For this review, use the dimensioned drawing (mm, ordinates from the lowest corner) and the shaded views. A direction names the side the tool comes from. Round coordinates to 2 decimals unless told otherwise and drop trailing zeros. Order: outer loops, then holes, each group sorted by start corner. A loop starts at its lowest first (then second) coordinate and runs counter-clockwise, first axis right, second up. Notation, with made-up numbers: M 63,26 L 105,26 A27 ccw 105,42 Z; hole C 63,-15 d2. An arc over 180 degrees is marked long. One line per item, written item: value. Start each with the question number.
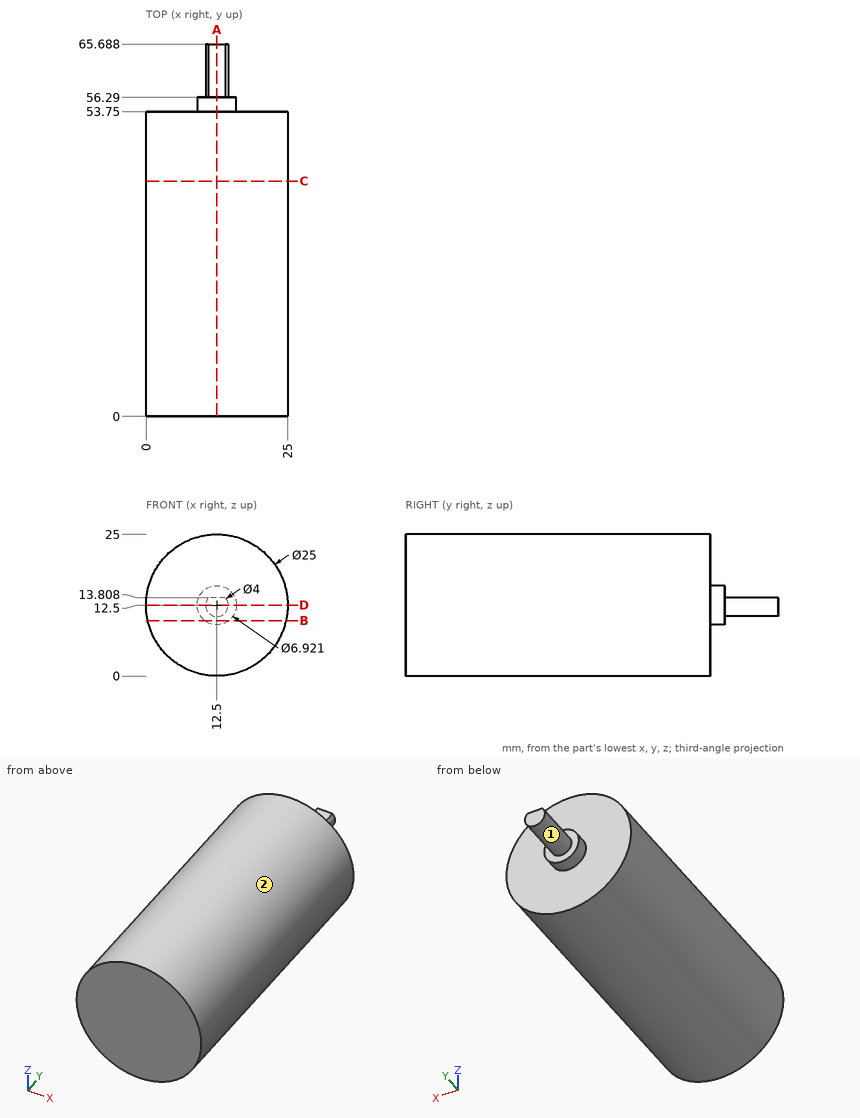
Item 1: Consider section A-A, the plane x = 12.5. Give the boundary of the cut face in (y, z), then the cut area to 3 significant figures.
Item 2: Clearance check with flat-ended pins moving along their axes: P1, Ø2, axis at y = 22.5, z = 8.5, coming from the -X side (1 decimal); P2, Ø2, axis at x = 10, y = 25.5, coming from the -Z side; P3, Ø8, axis at x = 20, y = 7, coming from the -Z side; P4, Ø6, axis at y = 28, z = 13, coming from the -X side. State where each tip first meets the part, or that it passes through.
Item 3: Consider section B-B, the plane z = 9.75. Give the boundary of the cut face in (x, y).
Item 4: Machinability: for the marked faces 1 and 2, which of the approach directions +Z, -Z, +X, -X, +Y, -Y give a long, thin tool a straight path to every point of the face, cutting with its end or side? Answer none if there is none.
Item 5: Wall thickness on L1, parallel to Y at x = 14, z = 1; L2, parallel to X at y = 37, z = 12; L3, parallel to Y at x = 9.5, z = 13.5: over which ranges is each line inside the solid? List them lowest first.
Item 6: Consider section C-C, the plane y = 41.5. Give the boundary of the cut face in (x, z).
Item 7: Consider section D-D, the plane z = 12.5. Give the boundary of the cut face in (x, y).
Computed:
1. outline: M 0,0 L 53.75,0 L 53.75,9.04 L 56.29,9.04 L 56.29,10.5 L 65.69,10.5 L 65.69,13.81 L 56.29,13.81 L 56.29,15.96 L 53.75,15.96 L 53.75,25 L 0,25 Z
1. area: 1,390 mm^2
2. P1: stops at x = 0.4
2. P2: stops at z = 0.09
2. P3: stops at z = 0.5
2. P4: stops at x = 0
3. outline: M 0.31,0 L 24.69,0 L 24.69,53.75 L 14.6,53.75 L 14.6,56.29 L 10.4,56.29 L 10.4,53.75 L 0.31,53.75 Z
4. face 1: +Y
4. face 2: +Y, -Y
5. L1: y = 0 to 53.75
5. L2: x = 0.01 to 24.99
5. L3: y = 0 to 56.29
6. outline: C 12.5,12.5 d25
7. outline: M 0,0 L 25,0 L 25,53.75 L 15.96,53.75 L 15.96,56.29 L 14.5,56.29 L 14.5,65.69 L 10.5,65.69 L 10.5,56.29 L 9.04,56.29 L 9.04,53.75 L 0,53.75 Z
